Read the model definition and answer for the solid it produces. Units are mm, in the model's axes. Face numbers are marked on the shaded views. A direction names the side the tool comes from. Coordinates: 2 decimals unless noted, no trailing zeros. Loops run counter-clockwise (first coordinate to the right, second up) from the corner with the lowest first, then second, coordinate; pieces in that order, holes last.
Q1. Which of the six approach directions +Z, -Z, +X, -X, +Y, -Y give full straight-line access (tool end or side, diameter ignored) to the marked faces 1, 2, 3, 4 and 5?
Q2. Section B-B (x = 2) is taken. Give the vertices of the cut face in (y, z) (3 decimals).
Q3. Section A-A (z = 5) is taken. Give the vertices of the cut face in (x, y) (3 decimals), then the cut area to 3 significant figures.
Q4. The mould has two halves that part along X. Classify the marked faces 6, 7 and 8: pulls with the +X half, pulls with the -X half, needs draft (parallel to the pull), parting line crosses it, or undercut.
Q5. Flat-ended cylindrical pins translate along their axes: P1, Ø5.5, axis at x = 2.5, z = 16, coming from the -Y side; P2, Ø5, axis at y = 6, z = 3, coming from the -X side; P3, Ø2, axis at y = 4.5, z = 4.5, coming from the -X side. Find the tip coordinate at first contact, or state that the pin passes through.
Q6. Section D-D (z = 15) is taken. Give the vertices of the cut face in (x, y).
Q7. Section C-C (y = 5) is taken. Give the vertices of the cut face in (x, z) (3 decimals), then the cut area to 3 significant figures.
Q8. Straight lines are drawn through the part: line 1 (X direction, y = 3.25, z = 5); line 2 (Y direction, x = 3.05, z = 5) (3 decimals); line 3 (Z direction, x = 2, y = 2.5). For each, find the intervals that lie inside material, in ascending order.
from build123d import *

# Parameters (mm, degrees)
SKETCH1_W           = 14.59
SKETCH1_H           = 10
BOSS_EXTRUDE1_DEPTH = 30
CUT_EXTRUDE1_DEPTH  = 3
SKETCH3_R           = 1.6
CUT_EXTRUDE2_DEPTH  = 10
CUT_EXTRUDE3_DEPTH  = 7
SKETCH5_R           = 2
BOSS_EXTRUDE2_DEPTH = 5
FILLET1_R           = 1
SKETCH6_R           = 2.075
CUT_EXTRUDE4_DEPTH  = 5
FILLET2_R           = 1


with BuildPart() as part:
    # Sketch1 → Boss-Extrude1 (new body)
    with BuildSketch(Plane.XY):
        with Locations((7.295, 5)):
            Rectangle(SKETCH1_W, SKETCH1_H)
    extrude(amount=BOSS_EXTRUDE1_DEPTH)

    # Sketch2 → Cut-Extrude1 (cut)
    with BuildSketch(Plane.XZ):
        with BuildLine():
            Line((0, 21), (3.507491981, 21))
            ThreePointArc((3.507491981, 21), (6.95, 15), (3.507491981, 9))
            Line((3.507491981, 9), (0, 9))
            Line((0, 9), (0, 21))
        make_face()
    extrude(amount=-CUT_EXTRUDE1_DEPTH, mode=Mode.SUBTRACT)

    # Sketch3 → Cut-Extrude2 (cut)
    with BuildSketch(Plane(origin=(0, 10, 0), x_dir=(1, 0, 0), z_dir=(0, 1, 0))):
        with Locations(Location((11.84, -5, 0), (0, 0, 270))):
            Circle(SKETCH3_R)
        with Locations(Location((11.84, -25, 0), (0, 0, 270))):
            Circle(SKETCH3_R)
    extrude(amount=-CUT_EXTRUDE2_DEPTH, mode=Mode.SUBTRACT)

    # Sketch4 → Cut-Extrude3 (cut)
    with BuildSketch(Plane(origin=(0, 10, 0), x_dir=(1, 0, 0), z_dir=(0, 1, 0))):
        with BuildLine():
            Line((0, -12), (0, -18))
            ThreePointArc((0, -18), (3, -15), (0, -12))
        make_face()
    extrude(amount=-CUT_EXTRUDE3_DEPTH, mode=Mode.SUBTRACT)

    # Sketch5 → Boss-Extrude2 (add)
    with BuildSketch(Plane.ZY):
        with Locations(Location((25, 5, 0), (0, 0, 180))):
            Circle(SKETCH5_R)
    extrude(amount=BOSS_EXTRUDE2_DEPTH)

    # Fillet1
    fillet1_edges = [part.edges().sort_by_distance(p)[0] for p in [
        (0, 5, 27),
    ]]
    fillet(fillet1_edges, radius=FILLET1_R)

    # Sketch6 → Cut-Extrude4 (cut)
    with BuildSketch(Plane.ZY):
        with Locations((5, 5)):
            Circle(SKETCH6_R)
    extrude(amount=-CUT_EXTRUDE4_DEPTH, mode=Mode.SUBTRACT)

    # Fillet2
    fillet2_edges = [part.edges().sort_by_distance(p)[0] for p in [
        (0, 5, 2.925),
    ]]
    fillet(fillet2_edges, radius=FILLET2_R)


solid = part.part
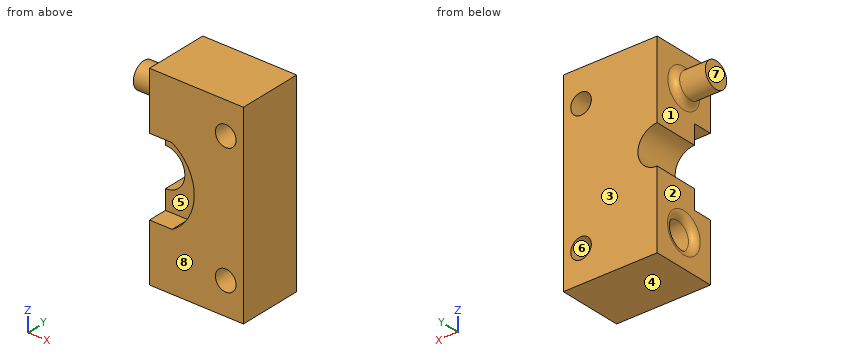
Numbers:
1. face 1: -X
1. face 2: -Z, -X, +Y, -Y
1. face 3: +Z, -Z, +X, -X, +Y
1. face 4: -Z, +X, -X, +Y, -Y
1. face 5: -X, -Y
2. outline: (0, 0) - (10, 0) - (10, 12.764) - (3, 12.764) - (3, 9) - (0, 9) - close; (0, 21) - (3, 21) - (3, 17.236) - (10, 17.236) - (10, 30) - (0, 30) - close; hole circle Ø4.15 at (5, 5)
3. outline: (0, 0) - (10.24, 0) - (10.24, 10) - (0, 10) - (0, 8.075) arc R1 ccw to (1, 7.075) - (5, 7.075) - (5, 2.925) - (1, 2.925) arc R1 ccw to (0, 1.925) - close; (13.44, 0) - (14.59, 0) - (14.59, 10) - (13.44, 10) - close
3. area: 92.7 mm2
4. face 6: undercut
4. face 7: pulls with the -X half
4. face 8: needs draft
5. P1: stops at y = 3
5. P2: stops at x = 0
5. P3: stops at x = 5
6. outline: (3, 3) - (6.95, 3) - (6.95, 0) - (14.59, 0) - (14.59, 10) - (3, 10) - close
7. outline: (-5, 23) - (-1, 23) arc R1 cw to (0, 22) - (0, 18) arc R3 cw to (0, 12) - (0, 8.075) arc R1 ccw to (1, 7.075) - (5, 7.075) - (5, 2.925) - (1, 2.925) arc R1 ccw to (0, 1.925) - (0, 0) - (14.59, 0) - (14.59, 30) - (0, 30) - (0, 28) arc R1 cw to (-1, 27) - (-5, 27) - close; hole circle Ø3.2 at (11.84, 5); hole circle Ø3.2 at (11.84, 25)
7. area: 407 mm2
8. line 1: x = 5 to 10.24, 13.44 to 14.59
8. line 2: y = 0 to 2.925, 7.075 to 10
8. line 3: z = 0 to 9, 21 to 30
